```python
from build123d import *

# Parameters (mm, degrees)
BOSS_EXTRUDE1_DEPTH      = 2.38125
BOSS_EXTRUDE2_DEPTH      = 27
BOSS_EXTRUDE2_DEPTH_BACK = 227


with BuildPart() as part:
    # Sketch1 → Boss-Extrude1 (new, symmetric)
    with BuildSketch(Plane.XY):
        Polygon((0, -127), (0, 127), (152.4, 17.892316301), (152.4, -121.807683699), align=None)
    extrude(amount=BOSS_EXTRUDE1_DEPTH, both=True)

    # Sketch4 → Boss-Extrude2 (add, two sides: drawn at the far end of the back side and taken through both)
    with BuildSketch(Plane(origin=(0, 100, 0), x_dir=(1, 0, 0), z_dir=(0, 1, 0)).offset(-BOSS_EXTRUDE2_DEPTH_BACK)):
        with BuildLine():
            Line((0, -2.38125), (0, 0))
            ThreePointArc((0, 0), (-0.01389267, -1.190949078), (-0.055563118, -2.38125))
            Line((-0.055563118, -2.38125), (0, -2.38125))
        make_face()
        with BuildLine():
            Line((0, 0), (0, 2.38125))
            Line((0, 2.38125), (-0.055563118, 2.38125))
            ThreePointArc((-0.055563118, 2.38125), (-0.01389267, 1.190949078), (0, 0))
        make_face()
    extrude(amount=BOSS_EXTRUDE2_DEPTH + BOSS_EXTRUDE2_DEPTH_BACK)


solid = part.part
```
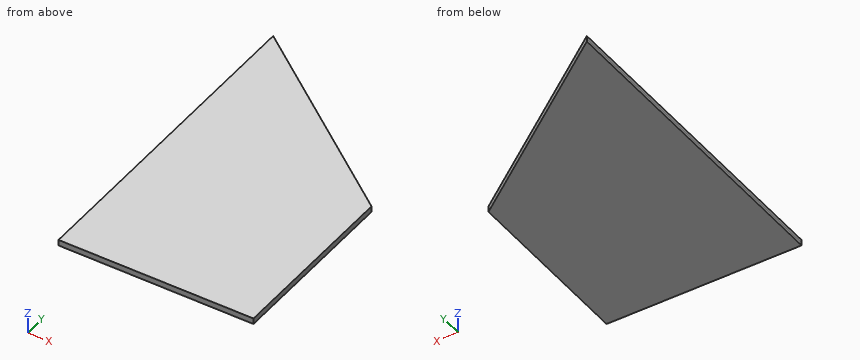
Source: CAD feature listing. Evaluate the final solid. Frame: model axes, mm. Round coordinates to 2 decimals unless told otherwise and drop trailing zeros. Order: outer loops, then holes, each group sorted by start corner. A loop starts at its lowest first (then second) coordinate and runs counter-clockwise, first axis right, second up. Notation, with made-up numbers: (81.5, 46) -> (114.5, 46) arc R13 ccw to (114.5, 58) -> close; hole circle Ø6 at (55.5, -38). An arc over 180 degrees is marked (long way). One line per item, written item: value. Start each with the question number.
Q1. Section query D-D (x = 75). Return the cut outline in (y, z).
Q2. Section query C-C (x = 32). Return the cut outline in (y, z).
Q3. Pin query (flat end, axial travel): pin 1 (1.5 mm diameter, centred on x = 81, z = 1, fed in from +Y); pin 2 (1.5 mm diameter, centred on x = 30.5, z = 1, fed in from -Y); pin 3 (1.5 mm diameter, centred on x = 35.5, z = 1.5, fed in from +Y). Return the tip coordinate at first contact, or that it passes through.
Q4. Section query A-A (y = 110.5). Return the cut outline in (x, z), plus the area to 3 significant figures.
Q5. Material intervals for probe 1 along X at (y, z) = (-99, -1.2); probe 2 along X at (y, z) = (89, -0.75); probe 3 along Y at (x, z) = (127, 1.5), sorted ascending.
Findings below:
1. outline: (-124.44, -2.38) -> (73.31, -2.38) -> (73.31, 2.38) -> (-124.44, 2.38) -> close
2. outline: (-125.91, -2.38) -> (104.09, -2.38) -> (104.09, 2.38) -> (-125.91, 2.38) -> close
3. pin 1: y = 69.55
3. pin 2: y = -125.99
3. pin 3: y = 102.12
4. outline: (-0.06, -2.38) -> (23.05, -2.38) -> (23.05, 2.38) -> (-0.06, 2.38) arc R51.05 cw to start
4. area: 110 mm²
5. probe 1: -0.01 to 152.4
5. probe 2: -0.01 to 53.08
5. probe 3: -122.67 to 36.08
